Geometry check sheet. Reference: the model listing, model coordinates, mm. Face numbers are marked on the shaded views. A direction names the side the tool comes from. Coordinates: 2 decimals unless noted, no trailing zeros. Write each loop counter-clockwise with the first axis right and the second up, starting at its lowest first coordinate (ties: lowest second). Pieces come first, ordered by that corner, then holes.
from build123d import *

# Parameters (mm, degrees)
SKETCH1_R                = 40
BOSS_EXTRUDE2_DEPTH      = 26
SKETCH3_R                = 23.5
CUT_EXTRUDE1_DEPTH       = 5
BOSS_EXTRUDE4_DEPTH      = 35
BOSS_EXTRUDE4_DEPTH_BACK = 35
SKETCH7_W                = 70
SKETCH7_H                = 16
SKETCH5_R                = 8.75
CUT_EXTRUDE9_DEPTH       = 10
SKETCH10_R               = 4
CUT_EXTRUDE10_DEPTH      = 9.4
SKETCH16_R               = 6.265
BOSS_EXTRUDE5_DEPTH      = 15
SKETCH18_R               = 4
CUT_EXTRUDE12_DEPTH      = 177.33290572
BOSS_EXTRUDE9_REACH      = 170.28
FILLET4_R                = 10
FILLET5_R                = 10
SKETCH4_R                = 1.5
CUT_EXTRUDE15_DEPTH      = 8
SKETCH25_R               = 6.265
BOSS_EXTRUDE10_DEPTH     = 15
BOSS_EXTRUDE11_DEPTH     = 15


with BuildPart() as part:
    # Sketch1 → Boss-Extrude2 (new body)
    with BuildSketch(Plane(origin=(0, 0, 0), x_dir=(1, 0, 0), z_dir=(0, 1, 0))):
        with Locations(Location((0, 0, 0), (0, 0, 90))):
            Circle(SKETCH1_R)
    extrude(amount=BOSS_EXTRUDE2_DEPTH)

    # Sketch3 → Cut-Extrude1 (cut)
    with BuildSketch(Plane.XZ):
        with Locations(Location((0, 0, 0), (0, 0, 270))):
            Circle(SKETCH3_R)
    extrude(amount=-CUT_EXTRUDE1_DEPTH, mode=Mode.SUBTRACT)

    # Sketch7 → Boss-Extrude4 (add, two sides: drawn at the far end of the back side and taken through both)
    with BuildSketch(Plane(origin=(0, 0, 0), x_dir=(0, 0, -1), z_dir=(1, 0, 0)).offset(-BOSS_EXTRUDE4_DEPTH_BACK)):
        with Locations((0, 18)):
            Rectangle(SKETCH7_W, SKETCH7_H)
    extrude(amount=BOSS_EXTRUDE4_DEPTH + BOSS_EXTRUDE4_DEPTH_BACK)

    # Sketch5 → Cut-Extrude9 (cut)
    with BuildSketch(Plane.XZ.offset(-5)):
        with Locations(Location((0, 0, 0), (0, 0, 270))):
            Circle(SKETCH5_R)
    extrude(amount=-CUT_EXTRUDE9_DEPTH, mode=Mode.SUBTRACT)

    # Sketch10 → Cut-Extrude10 (cut)
    with BuildSketch(Plane.XZ.offset(-15)):
        with Locations(Location((0, 0, 0), (0, 0, 270))):
            Circle(SKETCH10_R)
    extrude(amount=-CUT_EXTRUDE10_DEPTH, mode=Mode.SUBTRACT)

    # Sketch16 → Boss-Extrude5 (add)
    with BuildSketch(Plane.ZY.offset(35)):
        with BuildLine():
            Line((-35, 10), (-35, 26))
            Line((-35, 26), (14.400349673, 111.563915545))
            ThreePointArc((14.400349673, 111.563915545), (55.805794239, 122.658470979), (66.900349673, 81.253026413))
            Line((66.900349673, 81.253026413), (35, 26))
            Line((35, 26), (35, 10))
            Line((35, 10), (-35, 10))
        make_face()
        with Locations((0, 51.6)):
            Circle(SKETCH16_R, mode=Mode.SUBTRACT)
        with BuildLine():
            Line((27.5, 64.05), (42.5, 64.05))
            ThreePointArc((42.5, 64.05), (45.55, 61), (42.5, 57.95))
            Line((42.5, 57.95), (27.5, 57.95))
            ThreePointArc((27.5, 57.95), (24.45, 61), (27.5, 64.05))
        make_face(mode=Mode.SUBTRACT)
    boss_extrude5 = extrude(amount=BOSS_EXTRUDE5_DEPTH)

    # Mirror1: Boss-Extrude5 across plane
    add(boss_extrude5.mirror(Plane(origin=(0, 0, 0), x_dir=(0, 0, 1), z_dir=(1, 0, 0))))

    # Sketch18 → Cut-Extrude12 (cut, through all)
    with BuildSketch(Plane.ZY.offset(50)):
        with Locations((40.650349673, 96.408470979)):
            Circle(SKETCH18_R)
    extrude(amount=-CUT_EXTRUDE12_DEPTH, mode=Mode.SUBTRACT)

    # Sketch24 → Boss-Extrude9 (add, up to next)
    with BuildSketch(Plane(origin=(-35, 0, 0), x_dir=(0, 0, -1), z_dir=(1, 0, 0)), mode=Mode.PRIVATE) as boss_extrude9_sk1:
        Polygon((-40.196152423, 35), (-30, 35), (-30, 26), (-35, 26), align=None)
    boss_extrude9_tool1 = extrude(boss_extrude9_sk1.sketch, amount=BOSS_EXTRUDE9_REACH, mode=Mode.PRIVATE) - part.part
    add(boss_extrude9_tool1.solids().sort_by_distance((-35, 31.012908, 33.947102))[0])

    # Fillet4
    fillet4_edges = [part.edges().sort_by_distance(p)[0] for p in [
        (-35, 35, 35.098076211),
    ]]
    fillet(fillet4_edges, radius=FILLET4_R)

    # Fillet5
    fillet5_edges = [part.edges().sort_by_distance(p)[0] for p in [
        (35, 35, 35.098076211),
    ]]
    fillet(fillet5_edges, radius=FILLET5_R)

    # Sketch4 → Cut-Extrude15 (cut)
    with BuildSketch(Plane.XZ.offset(-5)):
        with Locations(Location((12, 0, 0), (0, 0, 270))):
            Circle(SKETCH4_R)
        with Locations(Location((0, -12, 0), (0, 0, 270))):
            Circle(SKETCH4_R)
        with Locations(Location((-12, 0, 0), (0, 0, 270))):
            Circle(SKETCH4_R)
        with Locations(Location((0, 12, 0), (0, 0, 270))):
            Circle(SKETCH4_R)
    extrude(amount=-CUT_EXTRUDE15_DEPTH, mode=Mode.SUBTRACT)

    # Sketch25 → Boss-Extrude10 (add)
    with BuildSketch(Plane.ZY.offset(-35)):
        with Locations((0, 51.6)):
            Circle(SKETCH25_R)
    extrude(amount=-BOSS_EXTRUDE10_DEPTH)

    # Sketch26 → Boss-Extrude11 (add)
    with BuildSketch(Plane.ZY.offset(-35)):
        with BuildLine():
            Line((27.5, 64.05), (42.5, 64.05))
            ThreePointArc((42.5, 64.05), (45.55, 61), (42.5, 57.95))
            Line((42.5, 57.95), (27.5, 57.95))
            ThreePointArc((27.5, 57.95), (24.45, 61), (27.5, 64.05))
        make_face()
    extrude(amount=-BOSS_EXTRUDE11_DEPTH)


solid = part.part
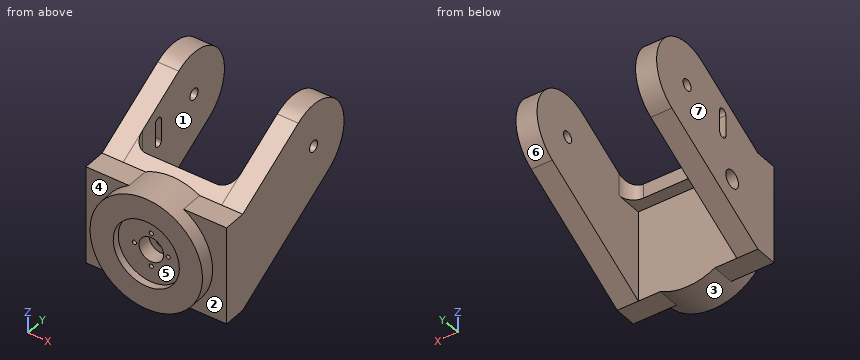
1. Thickness scan on line 1 along X through (y, z) = (8.75, 0); line 2 along X through (y, z) = (11, 0); line 3 along X through (y, z) = (47, 11). Record the ranges inside material, lowest first.
Computed values:
line 1: x = -40 to -13.5, -10.5 to -8.75, 8.75 to 10.5, 13.5 to 40
line 2: x = -50 to -13.5, -10.5 to -8.75, 8.75 to 10.5, 13.5 to 50
line 3: x = -50 to -35, 35 to 50
2. Access from +Z, -Z, +X, -X, +Y, -Y to the whole of each face (thin tool, end or side, straight path). Record for the marked faces 1, 2, 3 and 4.
Computed values:
face 1: -Z, +Y
face 2: +X, -Y
face 3: -Y
face 4: -X, -Y
3. Draft check along X on the marked faces 5, 6 and 7. Enter one of: released by +X, released by -X, zero draft, split by the parting line, or undercut.
Computed values:
face 5: undercut
face 6: zero draft
face 7: released by -X
4. Gauge pin test, flat ends, axial feed: pin 1 Ø5 at (x, y) = (-28.5, 18) entering from +Z; pin 2 Ø23 at (x, z) = (0, 0) entering from -Y; pin 3 Ø2 at (x, z) = (-4, 16.5) entering from +Y. Record the tip position at first contact, or that the pin passes through.
Computed values:
pin 1: stops at z = 35
pin 2: stops at y = 5
pin 3: stops at y = 26
5. Sectioned sample at D-D, the plane x = -16. Record the boundary of the cut face in (y, z).
Computed values:
outline: (0, -36.66) - (26, -36.66) - (26, 30) - (35, 30) - (35, 40.2) - (26, 35) - (26, 36.66) - (0, 36.66) - (0, 17.21) - (5, 17.21) - (5, -17.21) - (0, -17.21) - close
6. Sectioned sample at A-A, the plane y = 42. Record the boundary of the cut face in (x, z).
Computed values:
outline: (-50, -25.76) - (-35, -25.76) - (-35, 30) - (-34.54, 30) - (-34.54, 44.24) - (-50, 44.24) - close; (34.54, 30) - (35, 30) - (35, -25.76) - (50, -25.76) - (50, 44.24) - (34.54, 44.24) - close
7. Sectioned sample at C-C, the plane z = -31. Record the boundary of the cut face in (x, y).
Computed values:
outline: (-50, 10) - (-25.28, 10) - (-25.28, 0) - (25.28, 0) - (25.28, 10) - (50, 10) - (50, 32.93) - (35, 32.93) - (35, 26) - (-35, 26) - (-35, 32.93) - (-50, 32.93) - close
8. Sectioned sample at B-B, the plane y = 60.5. Record the boundary of the cut face in (x, z), and give its area (3 significant figures).
Computed values:
outline: (-50, -15.08) - (-35, -15.08) - (-35, 24.49) - (-50, 24.49) - close; (-50, 45.51) - (-35, 45.51) - (-35, 54.92) - (-50, 54.92) - close; (35, -15.08) - (50, -15.08) - (50, 54.92) - (35, 54.92) - close
area: 1,780 mm2
